Design review of the part built by this model. Coordinates are the model's own, in mm. A direction names the side the tool comes from. Give positions to 0.01 mm unless a question says otherwise; leave off trailing zeros. Write each loop counter-clockwise with the first axis right and the second up, starting at its lowest first coordinate (ties: lowest second). Pieces come first, ordered by that corner, then holes.
```python
from build123d import *

# Parameters (mm, degrees)
SKETCH3_R           = 1.5
BOSS_EXTRUDE3_DEPTH = 3
BOSS_EXTRUDE4_START = -25
BOSS_EXTRUDE4_DEPTH = 25
FILLET4_R           = 5
SKETCH9_W           = 42
SKETCH9_H           = 3
BOSS_EXTRUDE7_DEPTH = 30
FILLET6_R           = 5
FILLET7_R           = 5
SKETCH11_R          = 2.1
CUT_EXTRUDE2_DEPTH  = 30
SKETCH12_W          = 44.285709781
SKETCH12_H          = 8.726500344
CUT_EXTRUDE3_DEPTH  = 10
FILLET8_R           = 2.5


with BuildPart() as part:
    # Sketch3 → Boss-Extrude3 (new body)
    with BuildSketch(Plane.XY):
        with BuildLine():
            Line((-22.592834793, 16.50935751), (-6.092834793, 16.50935751))
            Line((-6.092834793, 16.50935751), (-6.092834793, 3.50935751))
            ThreePointArc((-6.092834793, 3.50935751), (-9.021766981, -3.561710302), (-16.092834793, -6.49064249))
            Line((-16.092834793, -6.49064249), (-38.092834793, -6.49064249))
            ThreePointArc((-38.092834793, -6.49064249), (-45.163902605, -3.561710302), (-48.092834793, 3.50935751))
            Line((-48.092834793, 3.50935751), (-48.092834793, 16.50935751))
            Line((-48.092834793, 16.50935751), (-31.592834793, 16.50935751))
            Line((-31.592834793, 16.50935751), (-22.592834793, 16.50935751))
        make_face()
        with Locations((-42.092834793, 11.50935751)):
            Circle(SKETCH3_R, mode=Mode.SUBTRACT)
        with Locations((-12.092834793, 11.50935751)):
            Circle(SKETCH3_R, mode=Mode.SUBTRACT)
    extrude(amount=BOSS_EXTRUDE3_DEPTH)

    # Sketch6 → Boss-Extrude4 (add)
    with BuildSketch(Plane.XY.offset(BOSS_EXTRUDE4_START)):
        with BuildLine():
            Line((-38.092834793, -6.49064249), (-16.092834793, -6.49064249))
            ThreePointArc((-16.092834793, -6.49064249), (-9.021766981, -3.561710302), (-6.092834793, 3.50935751))
            Line((-6.092834793, 3.50935751), (-48.092834793, 3.50935751))
            ThreePointArc((-48.092834793, 3.50935751), (-45.163902605, -3.561710302), (-38.092834793, -6.49064249))
        make_face()
    extrude(amount=BOSS_EXTRUDE4_DEPTH)

    # Fillet4
    fillet4_edges = [part.edges().sort_by_distance(p)[0] for p in [
        (-48.092834793, 16.50935751, 1.5),
        (-6.092834793, 16.50935751, 1.5),
    ]]
    fillet(fillet4_edges, radius=FILLET4_R)

    # Sketch9 → Boss-Extrude7 (add)
    with BuildSketch(Plane(origin=(0, 3.50935751, 0), x_dir=(1, 0, 0), z_dir=(0, 1, 0))):
        with Locations((-27.092834793, 23.5)):
            Rectangle(SKETCH9_W, SKETCH9_H)
    extrude(amount=-BOSS_EXTRUDE7_DEPTH)

    # Fillet6
    fillet6_edges = [part.edges().sort_by_distance(p)[0] for p in [
        (-6.092834793, -26.49064249, -23.5),
    ]]
    fillet(fillet6_edges, radius=FILLET6_R)

    # Fillet7
    fillet7_edges = [part.edges().sort_by_distance(p)[0] for p in [
        (-48.092834793, -26.49064249, -23.5),
    ]]
    fillet(fillet7_edges, radius=FILLET7_R)

    # Sketch11 → Cut-Extrude2 (cut)
    with BuildSketch(Plane(origin=(0, 0, -25), x_dir=(-1, 0, 0), z_dir=(0, 0, -1))):
        with Locations((9.592834793, -16.49064249)):
            Circle(SKETCH11_R)
        with Locations((44.592834793, -16.49064249)):
            Circle(SKETCH11_R)
        with BuildLine():
            Line((22.592834793, -24.49064249), (31.592834793, -24.49064249))
            ThreePointArc((31.592834793, -24.49064249), (27.092834793, -19.99064249), (22.592834793, -24.49064249))
        make_face()
    extrude(amount=-CUT_EXTRUDE2_DEPTH, mode=Mode.SUBTRACT)

    # Sketch12 → Cut-Extrude3 (cut)
    with BuildSketch(Plane(origin=(0, 0, -25), x_dir=(-1, 0, 0), z_dir=(0, 0, -1))):
        with Locations((28.235689684, -23.853892662)):
            Rectangle(SKETCH12_W, SKETCH12_H)
    extrude(amount=-CUT_EXTRUDE3_DEPTH, mode=Mode.SUBTRACT)

    # Fillet8
    fillet8_edges = [part.edges().sort_by_distance(p)[0] for p in [
        (-48.092834793, -19.49064249, -23.5),
        (-6.092834793, -19.49064249, -23.5),
    ]]
    fillet(fillet8_edges, radius=FILLET8_R)


solid = part.part
```
(1) Consider section B-B, the plane x = -12.5. Give the boundary of the cut face in (y, z), then the cut area to 3 significant figures.
Resolved:
outline: (-19.49, -25) - (3.51, -25) - (3.51, 0) - (10.07, 0) - (10.07, 3) - (-5.82, 3) - (-5.82, -22) - (-19.49, -22) - close; (12.95, 0) - (16.51, 0) - (16.51, 3) - (12.95, 3) - close
area: 333 mm2
(2) To check wall thickness, follow L1, parallel to Z at x = -26, y = -8.5; L2, parallel to Y at x = -23.5, z = -12; L3, parallel to Z at x = -43, y = 10. State the ranges of each line that lie inside material, in increasing order.
Resolved:
L1: z = -25 to -22
L2: y = -6.49 to 3.51
L3: z = 0 to 3
(3) Consider section D-D, the plane z = -16.25. Give the boundary of the cut face in (x, y).
Resolved:
outline: (-48.09, 3.51) arc R10 ccw to (-38.09, -6.49) - (-16.09, -6.49) arc R10 ccw to (-6.09, 3.51) - close
(4) Consider section A-A, the plane x = -29. Give the boundary of the cut face in (y, z).
Resolved:
outline: (-19.49, -25) - (3.51, -25) - (3.51, 0) - (16.51, 0) - (16.51, 3) - (-6.49, 3) - (-6.49, -22) - (-19.49, -22) - close
(5) Clearance check with flat-ended pins moving along their axes: P1, Ø1, axis at x = -19, z = -4, coming from the -Y side; P2, Ø5, axis at x = -9.59, y = -16.49, coming from the +Z side; P3, Ø1.5, axis at y = -1.5, z = -2, coming from the +X side. State where each tip first meets the part, or that it passes through.
Resolved:
P1: stops at y = -6.49
P2: stops at z = -22
P3: stops at x = -7.05
(6) Consider section C-C, the plane y = 6. Give the boundary of the cut face in (x, z).
Resolved:
outline: (-48.09, 0) - (-6.09, 0) - (-6.09, 3) - (-48.09, 3) - close
(7) Tool access review of faces 4 (the face through (-9.1, -3.64, -9.68)), 5 (the face through (-45.241, -3.484, -9.675)), 6 (the face through (-27, 3.509, -13)): name each direction out of +Z, -Z, +X, -X, +Y, -Y from which nothing blocks a thin tool from reaching the whole face with its end or side.
Resolved:
face 4: +Z, +X, -Y
face 5: +Z, -X, -Y
face 6: -Z, +X, -X, +Y
(8) Mouldability with a two-part tool opening along Y and no side actions: class faces 1 (the face through (-47.38, -18.74, -23.52)), 2 (the face through (-11.4, 10.18, 1.48)), 3 (the face through (-7.52, 15.01, 1.52)) as pulls with the +Y half, pulls with the -Y half, needs draft (parallel to the pull), parting line crosses it, or undercut.
Resolved:
face 1: pulls with the -Y half
face 2: undercut
face 3: pulls with the +Y half
